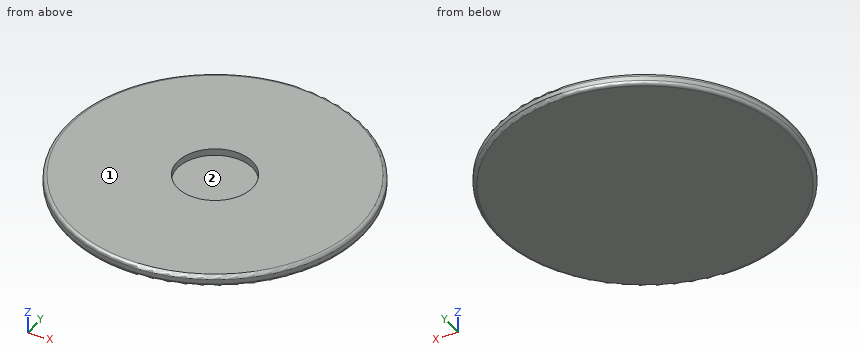
```python
from build123d import *

# Parameters (mm, degrees)
F0_R     = 6.5
F1_DEPTH = 0.5
F2_R     = 0.15
F3_R     = 1.65
F4_DEPTH = 0.3


# Not quite as in the source:
# - a feature names something its author has since deleted; it is built from what else it names


with BuildPart() as f1:
    # F0 (on Top) → F1 (new body)
    with BuildSketch(Plane.XY):
        Circle(F0_R)
    extrude(amount=F1_DEPTH)

    # F2
    f2_edges = [f1.edges().sort_by_distance(p)[0] for p in [
        (-6.5, 0, 0.5),
        (-6.5, 0, 0),
    ]]
    fillet(f2_edges, radius=F2_R)

    # F3 (on face) → F4 (cut)
    with BuildSketch(Plane.XY.offset(0.5)):
        Circle(F3_R)
    extrude(amount=-F4_DEPTH, mode=Mode.SUBTRACT)


solid = f1.part
```
The listing builds one solid part. Answer for the finished solid, in the listing's coordinates (mm). Face numbers are marked on the shaded views. Give positions to 0.01 mm unless a question says otherwise; leave off trailing zeros. Order: outer loops, then holes, each group sorted by start corner. A loop starts at its lowest first (then second) coordinate and runs counter-clockwise, first axis right, second up. Notation, with made-up numbers: (45, 0) -> (50, 0) arc R29 ccw to (50, 24) -> close; hole circle Ø10 at (-28.75, 39). An arc over 180 degrees is marked (long way). One line per item, written item: value.
1) Find the intervals of material crossed by line 1 (Y direction, x = 0, z = 0.3); line 2 (Z direction, x = 1.5, y = 0.5); line 3 (X direction, y = -1.5, z = 0.3), in increasing order.
Reported:
line 1: y = -6.5 to -1.65, 1.65 to 6.5
line 2: z = 0 to 0.2
line 3: x = -6.32 to -0.69, 0.69 to 6.32
2) Determine the mould class of the marked faces 1 and 2 for opening direction X: pulls with the +X half, pulls with the -X half, needs draft (parallel to the pull), parting line crosses it, or undercut.
Reported:
face 1: needs draft
face 2: undercut
3) A flat-ended cylindrical pin translates along its axis: P1, Ø6, axis at x = 1, y = 0.5, coming from the -Z side. Find the tip coordinate at first contact, or state that the pin passes through.
Reported:
P1: stops at z = 0
4) Find section A-A, the plane y = 0. Determine the outline of the cut face in (x, z).
Reported:
outline: (-6.5, 0.15) arc R0.15 ccw to (-6.35, 0) -> (6.35, 0) arc R0.15 ccw to (6.5, 0.15) -> (6.5, 0.35) arc R0.15 ccw to (6.35, 0.5) -> (1.65, 0.5) -> (1.65, 0.2) -> (-1.65, 0.2) -> (-1.65, 0.5) -> (-6.35, 0.5) arc R0.15 ccw to (-6.5, 0.35) -> close
